Design review of the part built by this model. Coordinates are the model's own, in mm. Coordinates: 2 decimals unless noted, no trailing zeros. Loops run counter-clockwise (first coordinate to the right, second up) from the corner with the lowest first, then second, coordinate; pieces in that order, holes last. Notation, with made-up numbers: (58.5, -39) -> (117.5, -39) arc R30 ccw to (117.5, -15) -> close; hole circle Ø10 at (16, -25.5). An arc over 180 degrees is marked (long way). Answer in a Markdown table with one row per item.
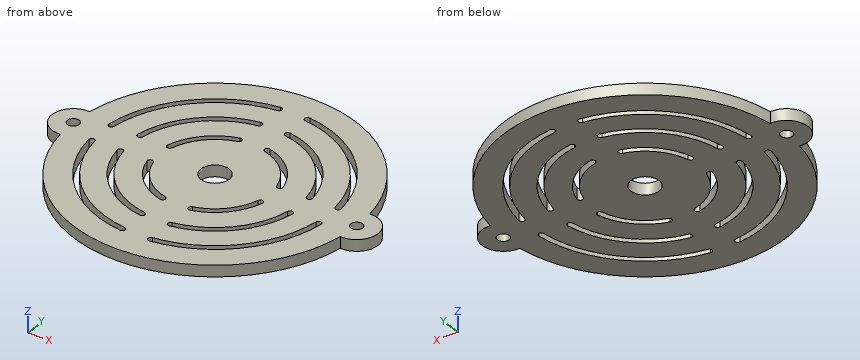
```python
from build123d import *

# Parameters (mm, degrees)
F0_R     = 2.08
F0_R_2   = 5
F1_DEPTH = 4


with BuildPart() as f1:
    # F0 (on Top) → F1 (new body)
    with BuildSketch(Plane.XY):
        with BuildLine():
            ThreePointArc((49.265581, 7.478732), (0, 49.83), (-49.265581, 7.478732))
            ThreePointArc((-49.265581, 7.478732), (-57.33, 0), (-49.265581, -7.478732))
            ThreePointArc((-49.265581, -7.478732), (0, -49.83), (49.265581, -7.478732))
            ThreePointArc((49.265581, -7.478732), (57.33, 0), (49.265581, 7.478732))
        make_face()
        with BuildLine():
            ThreePointArc((-5.124423, -40.865491), (-29.122569, -29.122569), (-40.865491, -5.124423))
            ThreePointArc((-40.865491, -5.124423), (-39.997684, -4.007771), (-38.881032, -4.875577))
            ThreePointArc((-38.881032, -4.875577), (-27.708355, -27.708355), (-4.875577, -38.881032))
            ThreePointArc((-4.875577, -38.881032), (-4.007771, -39.997684), (-5.124423, -40.865491))
        make_face(mode=Mode.SUBTRACT)
        with BuildLine():
            ThreePointArc((-5.165289, -30.82016), (-22.097087, -22.097087), (-30.82016, -5.165289))
            ThreePointArc((-30.82016, -5.165289), (-29.999205, -4.013755), (-28.84767, -4.834711))
            ThreePointArc((-28.84767, -4.834711), (-20.682873, -20.682873), (-4.834711, -28.84767))
            ThreePointArc((-4.834711, -28.84767), (-4.013755, -29.999205), (-5.165289, -30.82016))
        make_face(mode=Mode.SUBTRACT)
        with BuildLine():
            ThreePointArc((-20.333163, -5.25), (-19.614917, -4.031754), (-18.396671, -4.75))
            ThreePointArc((-18.396671, -4.75), (-13.435029, -13.435029), (-4.75, -18.396671))
            ThreePointArc((-4.75, -18.396671), (-4.031754, -19.614917), (-5.25, -20.333163))
            ThreePointArc((-5.25, -20.333163), (-14.849242, -14.849242), (-20.333163, -5.25))
        make_face(mode=Mode.SUBTRACT)
        with BuildLine():
            ThreePointArc((40.865491, -5.124423), (29.122569, -29.122569), (5.124423, -40.865491))
            ThreePointArc((5.124423, -40.865491), (4.007771, -39.997684), (4.875577, -38.881032))
            ThreePointArc((4.875577, -38.881032), (27.708355, -27.708355), (38.881032, -4.875577))
            ThreePointArc((38.881032, -4.875577), (39.997684, -4.007771), (40.865491, -5.124423))
        make_face(mode=Mode.SUBTRACT)
        with BuildLine():
            ThreePointArc((30.82016, -5.165289), (22.097087, -22.097087), (5.165289, -30.82016))
            ThreePointArc((5.165289, -30.82016), (4.013755, -29.999205), (4.834711, -28.84767))
            ThreePointArc((4.834711, -28.84767), (20.682873, -20.682873), (28.84767, -4.834711))
            ThreePointArc((28.84767, -4.834711), (29.999205, -4.013755), (30.82016, -5.165289))
        make_face(mode=Mode.SUBTRACT)
        with BuildLine():
            ThreePointArc((5.25, -20.333163), (4.031754, -19.614917), (4.75, -18.396671))
            ThreePointArc((4.75, -18.396671), (13.435029, -13.435029), (18.396671, -4.75))
            ThreePointArc((18.396671, -4.75), (19.614917, -4.031754), (20.333163, -5.25))
            ThreePointArc((20.333163, -5.25), (14.849242, -14.849242), (5.25, -20.333163))
        make_face(mode=Mode.SUBTRACT)
        with Locations((-49.83, 0)):
            Circle(F0_R, mode=Mode.SUBTRACT)
        Circle(F0_R_2, mode=Mode.SUBTRACT)
        with BuildLine():
            ThreePointArc((-20.333163, 5.25), (-14.849242, 14.849242), (-5.25, 20.333163))
            ThreePointArc((-5.25, 20.333163), (-4.031754, 19.614917), (-4.75, 18.396671))
            ThreePointArc((-4.75, 18.396671), (-13.435029, 13.435029), (-18.396671, 4.75))
            ThreePointArc((-18.396671, 4.75), (-19.614917, 4.031754), (-20.333163, 5.25))
        make_face(mode=Mode.SUBTRACT)
        with BuildLine():
            ThreePointArc((-30.82016, 5.165289), (-22.097087, 22.097087), (-5.165289, 30.82016))
            ThreePointArc((-5.165289, 30.82016), (-4.013755, 29.999205), (-4.834711, 28.84767))
            ThreePointArc((-4.834711, 28.84767), (-20.682873, 20.682873), (-28.84767, 4.834711))
            ThreePointArc((-28.84767, 4.834711), (-29.999205, 4.013755), (-30.82016, 5.165289))
        make_face(mode=Mode.SUBTRACT)
        with BuildLine():
            ThreePointArc((-40.865491, 5.124423), (-29.122569, 29.122569), (-5.124423, 40.865491))
            ThreePointArc((-5.124423, 40.865491), (-4.007771, 39.997684), (-4.875577, 38.881032))
            ThreePointArc((-4.875577, 38.881032), (-27.708355, 27.708355), (-38.881032, 4.875577))
            ThreePointArc((-38.881032, 4.875577), (-39.997684, 4.007771), (-40.865491, 5.124423))
        make_face(mode=Mode.SUBTRACT)
        with BuildLine():
            ThreePointArc((20.333163, 5.25), (19.614917, 4.031754), (18.396671, 4.75))
            ThreePointArc((18.396671, 4.75), (13.435029, 13.435029), (4.75, 18.396671))
            ThreePointArc((4.75, 18.396671), (4.031754, 19.614917), (5.25, 20.333163))
            ThreePointArc((5.25, 20.333163), (14.849242, 14.849242), (20.333163, 5.25))
        make_face(mode=Mode.SUBTRACT)
        with BuildLine():
            ThreePointArc((5.165289, 30.82016), (22.097087, 22.097087), (30.82016, 5.165289))
            ThreePointArc((30.82016, 5.165289), (29.999205, 4.013755), (28.84767, 4.834711))
            ThreePointArc((28.84767, 4.834711), (20.682873, 20.682873), (4.834711, 28.84767))
            ThreePointArc((4.834711, 28.84767), (4.013755, 29.999205), (5.165289, 30.82016))
        make_face(mode=Mode.SUBTRACT)
        with BuildLine():
            ThreePointArc((5.124423, 40.865491), (29.122569, 29.122569), (40.865491, 5.124423))
            ThreePointArc((40.865491, 5.124423), (39.997684, 4.007771), (38.881032, 4.875577))
            ThreePointArc((38.881032, 4.875577), (27.708355, 27.708355), (4.875577, 38.881032))
            ThreePointArc((4.875577, 38.881032), (4.007771, 39.997684), (5.124423, 40.865491))
        make_face(mode=Mode.SUBTRACT)
        with Locations((49.83, 0)):
            Circle(F0_R, mode=Mode.SUBTRACT)
    extrude(amount=F1_DEPTH)


solid = f1.part
```
(1) Take a section at B-B on y = 33. Give the boundary of the cut face in (x, z).
Evaluation:
| item | result |
|---|---|
| outline | (-37.34, 0) -> (-24.64, 0) -> (-24.64, 4) -> (-37.34, 4) -> close; (-21.13, 0) -> (21.13, 0) -> (21.13, 4) -> (-21.13, 4) -> close; (24.64, 0) -> (37.34, 0) -> (37.34, 4) -> (24.64, 4) -> close |
(2) Take a section at A-A on x = 13.5. Give the boundary of the cut face in (y, z), and give its area (3 significant figures).
Evaluation:
| item | result |
|---|---|
| outline | (-47.97, 0) -> (-38.91, 0) -> (-38.91, 4) -> (-47.97, 4) -> close; (-36.79, 0) -> (-28.18, 0) -> (-28.18, 4) -> (-36.79, 4) -> close; (-25.95, 0) -> (-16.09, 0) -> (-16.09, 4) -> (-25.95, 4) -> close; (-13.37, 0) -> (13.37, 0) -> (13.37, 4) -> (-13.37, 4) -> close; (16.09, 0) -> (25.95, 0) -> (25.95, 4) -> (16.09, 4) -> close; (28.18, 0) -> (36.79, 0) -> (36.79, 4) -> (28.18, 4) -> close; (38.91, 0) -> (47.97, 0) -> (47.97, 4) -> (38.91, 4) -> close |
| area | 327 mm² |
(3) Take a section at D-D on y = 22. Give the boundary of the cut face in (x, z), and give its area (3 significant figures).
Evaluation:
| item | result |
|---|---|
| outline | (-44.71, 0) -> (-34.82, 0) -> (-34.82, 4) -> (-44.71, 4) -> close; (-32.43, 0) -> (-22.19, 0) -> (-22.19, 4) -> (-32.43, 4) -> close; (-19.28, 0) -> (19.28, 0) -> (19.28, 4) -> (-19.28, 4) -> close; (22.19, 0) -> (32.43, 0) -> (32.43, 4) -> (22.19, 4) -> close; (34.82, 0) -> (44.71, 0) -> (44.71, 4) -> (34.82, 4) -> close |
| area | 315 mm² |
(4) Take a section at C-C on y = 10. Give the boundary of the cut face in (x, z).
Evaluation:
| item | result |
|---|---|
| outline | (-48.82, 0) -> (-39.95, 0) -> (-39.95, 4) -> (-48.82, 4) -> close; (-37.89, 0) -> (-29.61, 0) -> (-29.61, 4) -> (-37.89, 4) -> close; (-27.49, 0) -> (-18.47, 0) -> (-18.47, 4) -> (-27.49, 4) -> close; (-16.16, 0) -> (16.16, 0) -> (16.16, 4) -> (-16.16, 4) -> close; (18.47, 0) -> (27.49, 0) -> (27.49, 4) -> (18.47, 4) -> close; (29.61, 0) -> (37.89, 0) -> (37.89, 4) -> (29.61, 4) -> close; (39.95, 0) -> (48.82, 0) -> (48.82, 4) -> (39.95, 4) -> close |
(5) For pin 1 (2 mm diameter, centred on x = -16.5, y = 14.5, fed in from -Z); pin 2 (1.5 mm diameter, centred on x = 27, z = 3, fed in from -Y), all flat-tipped, find the tip position at first contact; note any pin that passes through.
Evaluation:
| item | result |
|---|---|
| pin 1 | stops at z = 0 |
| pin 2 | stops at y = -42.36 |
(6) To check wall thickness, follow probe 1 along Y at (x, z) = (49.83, 1.7); probe 2 along Y at (x, z) = (0, 1.95); probe 3 along X at (y, z) = (-21, 2.55). State the ranges of each line that lie inside material, in increasing order.
Evaluation:
| item | result |
|---|---|
| probe 1 | y = -7.5 to -2.08, 2.08 to 7.5 |
| probe 2 | y = -49.83 to -5, 5 to 49.83 |
| probe 3 | x = -45.19 to -35.43, -33.08 to -23.14, -20.36 to 20.36, 23.14 to 33.08, 35.43 to 45.19 |
